Autodesk Inventor part; units mm, degrees
ref_plane "YZ Plane" through (0, 0, 0) normal (1, 0, 0) x (0, 1, 0)
ref_plane "XZ Plane" through (0, 0, 0) normal (0, 1, 0) x (-1, 0, 0)
ref_plane "XY Plane" through (0, 0, 0) normal (0, 0, 1) x (1, 0, 0)
ref_plane "Work Plane2" through (30.8055, -26.6615, 12.7) normal (0, 0, 1) x (1, 0, 0)
sketch "Sketch2" plane through (30.8055, -26.6615, 12.7) normal (0, 0, 1) x (1, 0, 0)
  circle A0 centre (-30.8055, 26.6615) radius 13
  dimension "d0" = 26
extrude "Extrusion1" add sketch "Sketch2" along normal blind 12
sketch "Sketch5" plane through (0, 0, 12.7) normal (0, 0, -1) x (-1, 0, 0)
  line L0 (-4.7625, 7.9375) -> (4.7509, 7.9375)
  line L1 (4.7509, 7.9375) -> (4.7509, 4.7625)
  line L2 (4.7509, 4.7625) -> (-4.7625, 4.7625)
  line L3 (-4.7625, 4.7625) -> (-4.7625, 7.9375)
  line L4 (-4.7625, 1.5875) -> (4.7509, 1.5875)
  line L5 (4.7509, 1.5875) -> (4.7509, -1.5875)
  line L6 (4.7509, -1.5875) -> (-4.7625, -1.5875)
  line L7 (-4.7625, -1.5875) -> (-4.7625, 1.5875)
  line L8 (-4.7672, -4.7625) -> (4.7509, -4.7625)
  line L9 (4.7509, -4.7625) -> (4.7509, -7.9375)
  line L10 (4.7509, -7.9375) -> (-4.7672, -7.9375)
  line L11 (-4.7672, -7.9375) -> (-4.7672, -4.7625)
  point P0 (0, 0)
extrude "Extrusion4" add sketch "Sketch5" along normal blind 12.7
sketch "Sketch8" plane through (-4.7509, -7.9375, 12.7) normal (0, -1, 0) x (1, 0, 0)
  circle A0 centre (3.9555, -7.9375) radius 1.5875
  line L0 (9.5181, 0) -> (9.5181, -12.7)
  point P0 (4.7509, -12.7)
  dimension "d17" = 5.5626
extrude "Extrusion7" cut sketch "Sketch8" against normal blind 25.4
properties part number "Swing_Joint"
Work out the finished part from the listing and answer in its coordinate system (mm). A direction names the side the tool comes from. Coordinates: 2 decimals unless noted, no trailing zeros. Loops run counter-clockwise (first coordinate to the right, second up) from the corner with the lowest first, then second, coordinate; pieces in that order, holes last. Notation, with made-up numbers: (68.25, -7.75) -> (72.25, -7.75) arc R8 ccw to (72.25, 2.25) -> close; hole circle Ø6 at (59, -31). An arc over 180 degrees is marked (long way). Answer as CSV lines item,"result".
1) The part is cut by section D-D (z = 16.25). Give the vertices of the cut face in (x, y).
A:
outline,"circle Ø26 at (0, 0)"
2) The part is cut by section A-A (z = 7.75). Give the vertices of the cut face in (x, y).
A:
outline,"(-4.75, -7.94) -> (4.77, -7.94) -> (4.77, -4.76) -> (-4.75, -4.76) -> close; (-4.75, -1.59) -> (4.76, -1.59) -> (4.76, 1.59) -> (-4.75, 1.59) -> close; (-4.75, 4.76) -> (4.76, 4.76) -> (4.76, 7.94) -> (-4.75, 7.94) -> close"
3) For faces 1 (the face through (-0.1, -1.588, 6.4)), 2 (the face through (0.1, 7.938, 6.4)), 3 (the face through (-4.751, 6, 6)), determine the directions among +Z, -Z, +X, -X, +Y, -Y from which every point of the face is accessible in a straight line to the end or side of a thin tool.
A:
face 1,"-Z, +X, -X"
face 2,"-Z, +X, -X, +Y"
face 3,"-Z, -X, +Y, -Y"
4) The part is cut by section B-B (y = 0). Give the vertices of the cut face in (x, z) (1 decimal).
A:
outline,"(-13, 12.7) -> (-4.8, 12.7) -> (-4.8, 0) -> (4.8, 0) -> (4.8, 12.7) -> (13, 12.7) -> (13, 24.7) -> (-13, 24.7) -> close; hole circle Ø3.2 at (-0.8, 4.8)"
5) The part is cut by section C-C (x = 0). Give the vertices of the cut face in (y, z).
A:
outline,"(-13, 12.7) -> (-7.94, 12.7) -> (-7.94, 6.14) -> (-4.76, 6.14) -> (-4.76, 12.7) -> (-1.59, 12.7) -> (-1.59, 6.14) -> (1.59, 6.14) -> (1.59, 12.7) -> (4.76, 12.7) -> (4.76, 6.14) -> (7.94, 6.14) -> (7.94, 12.7) -> (13, 12.7) -> (13, 24.7) -> (-13, 24.7) -> close; (-7.94, 0) -> (-4.76, 0) -> (-4.76, 3.39) -> (-7.94, 3.39) -> close; (-1.59, 0) -> (1.59, 0) -> (1.59, 3.39) -> (-1.59, 3.39) -> close; (4.76, 0) -> (7.94, 0) -> (7.94, 3.39) -> (4.76, 3.39) -> close"
6) Straight lines are drawn through the part: probe 1 along Y at (x, z) = (1, 5.75); probe 2 along Z at (x, y) = (9.25, 4.25); probe 3 along Y at (x, z) = (1.75, 16.5). For each, find the intervals that lie inside material, in ascending order.
A:
probe 1,"y = -7.94 to -4.76, -1.59 to 1.59, 4.76 to 7.94"
probe 2,"z = 12.7 to 24.7"
probe 3,"y = -12.88 to 12.88"
7) For a pull along Z with two mould halves and no side action, classify faces 4 (the face through (0, 0, 0)), 5 (the face through (0.06, -0.02, 6.1)), 6 (the face through (0.1, -4.762, 6.4)), 7 (the face through (0, 0, 24.7)) as released by +Z, released by -Z, zero draft, split by the parting line, or undercut.
A:
face 4,"released by -Z"
face 5,"undercut"
face 6,"zero draft"
face 7,"released by +Z"
8) Flat-ended cylindrical pins translate along their axes: pin 1 (2.5 mm diameter, centred on y = -6.5, z = 7, fed in from -X); pin 2 (10 mm diameter, centred on x = 9.5, z = 3, fed in from -Y); pin 3 (12 mm diameter, centred on y = -6.5, z = 15, fed in from -X); pin 4 (1.9 mm diameter, centred on x = -0.8, z = 4.76, fed in from -Y). Find the tip coordinate at first contact, or state that the pin passes through.
A:
pin 1,"stops at x = -4.75"
pin 2,"stops at y = -7.94"
pin 3,"stops at x = -12.99"
pin 4,"passes through"
